Verification items for this drawing (mm, ordinates from the low corner). A direction names the side the tool comes from. Round coordinates to 2 decimals unless told otherwise and drop trailing zeros. Order: outer loops, then holes, each group sorted by start corner. A loop starts at its lowest first (then second) coordinate and runs counter-clockwise, first axis right, second up. Notation, with made-up numbers: M 85.5,88.5 L 123.5,88.5 A26 cw 123.5,127.5 Z; hole C -37,44.25 d9. An arc over 180 degrees is marked long. Return JSON: item names as keys, results as strings. Group by question number.
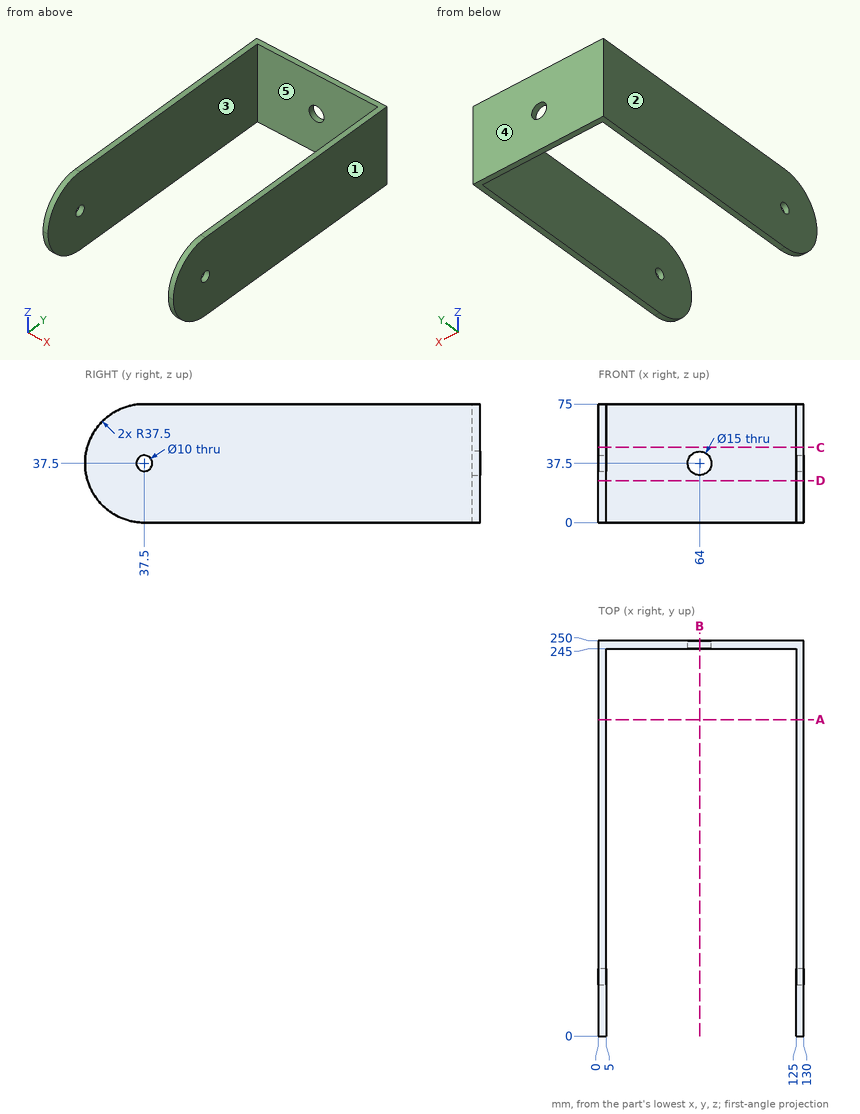
Q1. Section check B-B on x = 64. Record the cut outline in (y, z), plus the area to 3 significant figures.
Q2. Release check for a two-part mould opening along X. For the marked faces 1, 2 and 3 record: +X half, -X half, draft (parallel to the pull), parting line (faces both ways), or undercut.
Q3. Material ranges on line 1 along X through (y, z) = (247, 37); line 2 along X through (y, z) = (45, 66.5); line 3 along Z through (x, y) = (3, 37) (1 decimal), recorded low to high.
Q4. Section check C-C on z = 47.5. Record the cut outline in (x, y), plus the area to 3 significant figures.
Q5. Depth check by flat-ended pin: pin 1 Ø19.5 at (x, z) = (64, 37.5) entering from -Y; pin 2 Ø13 at (y, z) = (37.5, 37.5) entering from -X. Enter the tip coordinate at first touch or a pass-through.
Q6. Section check A-A on y = 200. Record the cut outline in (x, z).
Q7. Set-up check for the marked faces 4 and 5: record each of +Z, -Z, +X, -X, +Y, -Y from which the full face is reachable in a straight line by a thin tool's end or side.
Q8. Section check D-D on z = 26.5. Record the cut outline in (x, y).
Geometry check:
{
 "1": {"outline": "M 245,0 L 250,0 L 250,30 L 245,30 Z; M 245,45 L 250,45 L 250,75 L 245,75 Z", "area": "300 mm^2"},
 "2": {"face 1": "+X half", "face 2": "-X half", "face 3": "undercut"},
 "3": {"line 1": "x = 0 to 56.52, 71.48 to 130", "line 2": "x = 0 to 5, 125 to 130", "line 3": "z = 0 to 32.5, 42.5 to 75"},
 "4": {"outline": "M 0,1.36 L 5,1.36 L 5,245 L 125,245 L 125,1.36 L 130,1.36 L 130,250 L 0,250 Z", "area": "3,090 mm^2"},
 "5": {"pin 1": "stops at y = 245", "pin 2": "stops at x = 0"},
 "6": {"outline": "M 0,0 L 5,0 L 5,75 L 0,75 Z; M 125,0 L 130,0 L 130,75 L 125,75 Z"},
 "7": {"face 4": "+Z, -Z, +X, -X, +Y", "face 5": "+Z, -Z, -Y"},
 "8": {"outline": "M 0,1.65 L 5,1.65 L 5,245 L 125,245 L 125,1.65 L 130,1.65 L 130,250 L 0,250 Z"}
}
